```python
from build123d import *

# Parameters (mm, degrees)
SKETCH1_W           = 15
SKETCH1_H           = 4
SKETCH1_W_2         = 10
SKETCH1_H_2         = 128
SKETCH1_R           = 1.4
SKETCH1_R_2         = 1.5
BOSS_EXTRUDE1_DEPTH = 3


with BuildPart() as part:
    # Sketch1 → Boss-Extrude1 (new body)
    # profile 1 of 2: a face of its own
    with BuildSketch(Plane(origin=(0, 0, 0), x_dir=(1, 0, 0), z_dir=(0, 1, 0))):
        with Locations((42.376726578, -144.989284628)):
            Rectangle(SKETCH1_W, SKETCH1_H)
    # profile 2 of 2: a face of its own
    with BuildSketch(Plane(origin=(0, 0, 0), x_dir=(1, 0, 0), z_dir=(0, 1, 0))):
        with Locations((42.376726578, -78.989284628)):
            Rectangle(SKETCH1_W_2, SKETCH1_H_2)
        with Locations(Location((42.376726578, -22.989284628, 0), (0, 0, 270))):
            Circle(SKETCH1_R, mode=Mode.SUBTRACT)
        with Locations(Location((42.376726578, -32.989284628, 0), (0, 0, 270))):
            Circle(SKETCH1_R, mode=Mode.SUBTRACT)
        with Locations(Location((42.376726578, -136.989284628, 0), (0, 0, 270))):
            Circle(SKETCH1_R_2, mode=Mode.SUBTRACT)
        with Locations(Location((42.376726578, -84.989284628, 0), (0, 0, 270))):
            Circle(SKETCH1_R_2, mode=Mode.SUBTRACT)
        with Locations(Location((42.376726578, -74.989284628, 0), (0, 0, 270))):
            Circle(SKETCH1_R_2, mode=Mode.SUBTRACT)
    extrude(amount=BOSS_EXTRUDE1_DEPTH)


solid = part.part
```
Build history of the part. All positions in model axes, mm. A direction names the side the tool comes from. Round coordinates to 2 decimals unless told otherwise and drop trailing zeros. Write each loop counter-clockwise with the first axis right and the second up, starting at its lowest first coordinate (ties: lowest second). Pieces come first, ordered by that corner, then holes. Notation, with made-up numbers: (49.25, 9) - (99.25, 9) arc R11 ccw to (99.25, 23) - close; hole circle Ø10 at (29, -19.5). An arc over 180 degrees is marked (long way). Write each question's results on one line, items separated by ' | '. Start each with the question number.
Item 1: Saw through at C-C (x = 36). Write the cut outline in (y, z).
Item 2: Mould opens along Z. For faces 1 (the face through (42, 1, 14.989)), 2 (the face through (43.64, 1.48, 75.8)), 3 (the face through (47.377, 1, 80)) say: pulls with the +Z half, pulls with the -Z half, needs draft (parallel to the pull), parting line crosses it, or undercut.
Item 3: Wall check: L1, parallel to X at y = 1.9, z = 73; L2, parallel to Z at x = 36.75, y = 2.85; L3, parallel to X at y = 0.1, z = 32.5 (3 decimals). Give the ranges that are in metal, low to high. Write a range as [from, to].
Item 4: Drop flat-ended pins along their axis: P1, Ø1.2, axis at x = 49, y = 1, coming from the -Z side; P2, Ø1.5, axis at y = 1.5, z = 124, coming from the -X side; P3, Ø4.5, axis at x = 42.38, z = 22.99, coming from the +Y side. Give the stop position or say it passes through.
Item 5: Which spindle directions (+Z, -Z, +X, -X, +Y, -Y) get a long thin tool onto all of the face, cutting with end or side? Do faces 4 (the face through (37.377, 1, 80)), 5 (the face through (49, 1, 142.989)), 6 (the face through (41.01, 1.48, 22.69)). Say none if no direction does.
Item 6: Saw through at A-A (z = 137). Write the cut outline in (x, y), and give its area (3 significant figures).
Item 7: Saw through at D-D (z = 91.5). Write the cut outline in (x, y).
Item 8: Saw through at B-B (y = 1.3). Write the cut outline in (x, z), and give its area (3 significant figures).
Results are:
1) outline: (0, 142.99) - (3, 142.99) - (3, 146.99) - (0, 146.99) - close
2) face 1: pulls with the -Z half | face 2: undercut | face 3: needs draft
3) L1: x = [37.38, 47.38] | L2: z = [142.99, 146.99] | L3: x = [37.377, 41.065], [43.688, 47.377]
4) P1: stops at z = 142.99 | P2: stops at x = 37.38 | P3: stops at y = 3
5) face 4: -Z, -X, +Y, -Y | face 5: -Z, +X, +Y, -Y | face 6: +Y, -Y
6) outline: (37.38, 0) - (40.88, 0) - (40.88, 3) - (37.38, 3) - close; (43.88, 0) - (47.38, 0) - (47.38, 3) - (43.88, 3) - close | area: 21.0 mm²
7) outline: (37.38, 0) - (47.38, 0) - (47.38, 3) - (37.38, 3) - close
8) outline: (34.88, 142.99) - (37.38, 142.99) - (37.38, 14.99) - (47.38, 14.99) - (47.38, 142.99) - (49.88, 142.99) - (49.88, 146.99) - (34.88, 146.99) - close; hole circle Ø3 at (42.38, 74.99); hole circle Ø3 at (42.38, 84.99); hole circle Ø3 at (42.38, 136.99); hole circle Ø2.8 at (42.38, 22.99); hole circle Ø2.8 at (42.38, 32.99) | area: 1,310 mm²
